Input: part model. Units: mm. Frame: model coordinates. Face numbers are marked on the shaded views. A direction names the side the tool comes from. Round coordinates to 2 decimals unless told otherwise and drop trailing zeros. Loops run counter-clockwise (first coordinate to the right, second up) from the corner with the lowest first, then second, coordinate; pieces in that order, holes last. Notation, with made-up numbers: (66.5, -12.5) -> (72.5, -12.5) arc R16 ccw to (72.5, 13.5) -> close; hole circle Ø3 at (-13, -25). An arc over 180 degrees is marked (long way). Answer as a JSON object with one key per item and string values. Group by question number.
Item 1: Pin query (flat end, axial travel): pin 1 (15 mm diameter, centred on y = 72, z = 8.5, fed in from -X); pin 2 (9 mm diameter, centred on x = -126.5, z = 16, fed in from +Y). Return the tip coordinate at first contact, or that it passes through.
Item 2: Material intervals for line 1 (Y direction, x = 7, z = 116.5); line 2 (X direction, y = -1, z = 238.5); line 3 (Z direction, x = 8.5, y = 90), sorted ascending. Write a range as [from, to].
Item 3: Section query C-C on z = 450. Return loops of the section in (x, y), and give its area (3 significant figures).
Item 4: Set-up query: the marked faces 1 and 2. Return all of +Z, -Z, +X, -X, +Y, -Y with unobstructed straight access to the full face (end or side cutting, diameter ignored); none if empty.
Item 5: Section query A-A on x = -6. Return loops of the section in (y, z), and give its area (3 significant figures).
Item 6: Section query B-B on y = 122. Return loops of the section in (x, z), and give its area (3 significant figures).
from build123d import *

# Parameters (mm, degrees)
F0_W     = 42.2
F0_H     = 30
F1_DEPTH = 800
F2_DEPTH = 30


with BuildPart() as f1:
    # F0 (on Top) → F1 (new body)
    with BuildSketch(Plane.XY):
        Rectangle(F0_W, F0_H)
    extrude(amount=F1_DEPTH)

    # F0 (on Top) → F2 (join)
    with BuildSketch(Plane.XY):
        Polygon((-171.1, -15), (-21.1, -15), (-21.1, 15), (-21.1, 27.2), (-171.1, 27.2), align=None)
        Polygon((-21.1, 15), (21.1, 15), (21.1, 165), (-21.1, 165), (-21.1, 27.2), align=None)
    extrude(amount=F2_DEPTH)


solid = f1.part
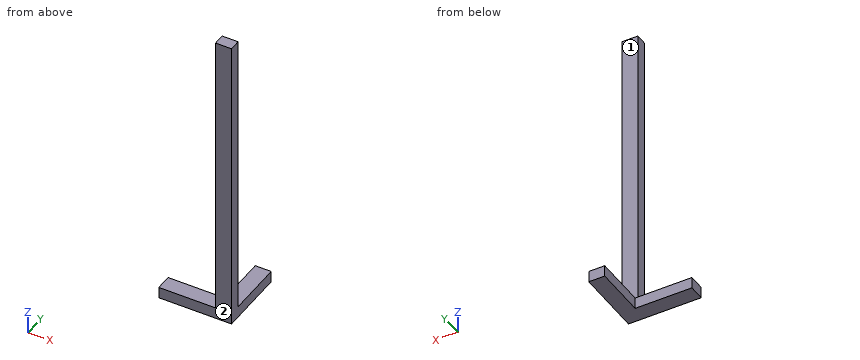
Solved:
{
 "1": {"pin 1": "x = -21.1", "pin 2": "y = 27.2"},
 "2": {"line 1": "[-15, 15]", "line 2": "[-21.1, 21.1]", "line 3": "[0, 30]"},
 "3": {"outline": "(-21.1, -15) -> (21.1, -15) -> (21.1, 15) -> (-21.1, 15) -> close", "area": "1,270 mm²"},
 "4": {"face 1": "+Z, +X, -X, +Y", "face 2": "+Z, -Z, +X, -X, -Y"},
 "5": {"outline": "(-15, 0) -> (165, 0) -> (165, 30) -> (15, 30) -> (15, 800) -> (-15, 800) -> close", "area": "28,500 mm²"},
 "6": {"outline": "(-21.1, 0) -> (21.1, 0) -> (21.1, 30) -> (-21.1, 30) -> close", "area": "1,270 mm²"}
}
